The listing builds one solid part. Answer for the finished solid, in the listing's coordinates (mm). A direction names the side the tool comes from. Give positions to 0.01 mm unless a question says otherwise; leave off trailing zeros. Order: outer loops, then holes, each group sorted by start corner. A loop starts at its lowest first (then second) coordinate and runs counter-clockwise, first axis right, second up. Notation, with made-up numbers: (19, 2.5) - (64, 2.5) arc R15 cw to (64, 29.5) - close; hole circle Ø11 at (-33, -10.5). An arc over 180 degrees is marked (long way). Write each question's results on one line, items separated by ' | '. Start each with the question number.
1. Find the intervals of material crossed by L1, parallel to Z at x = -15.5, y = 0; L2, parallel to Y at x = -14, z = 1.5, in increasing order.
2. Which of the six approach directions +Z, -Z, +X, -X, +Y, -Y give full straight-line access (tool end or side, diameter ignored) to faces 4 (the face through (-61.5, 4, 12)), 5 (the face through (-76.014, -3.685, 11.701)), 6 (the face through (0, 0, 0))?
3. Section A-A (z = 0) is taken. Give the vertices of the cut face in (x, y).
4. Flat-ended cylindrical pins translate along their axes: pin 1 (5 mm diameter, centred on x = -77, y = 1.5, fed in from +Z); pin 2 (1 mm diameter, centred on x = -13.5, y = 1, fed in from +Z); pin 3 (3 mm diameter, centred on y = 5.5, z = 11, fed in from -X). Find the tip coordinate at first contact, or state that the pin passes through.
5. Section D-D (x = -120) is taken. Give the vertices of the cut face in (y, z).
6. Section C-C (x = -13) is taken. Give the vertices of the cut face in (y, z).
7. Determine the mould class of faces 1 (the face through (-64.035, 10.648, -13.887)), 2 (the face through (-80.56, -0.53, -11.99)), 3 (the face through (-8.16, 9.43, -2.09)) for opening direction X: released by +X, released by -X, zero draft, split by the parting line, or undercut.
from build123d import *

# Parameters (mm, degrees)
F2_SIZE2 = 2
F2_SIZE  = 2
F3_SIZE2 = 2.5
F3_SIZE  = 2.5


with BuildPart() as f1:
    # F0 (on Front) → F1 (revolve)
    with BuildSketch(Plane.XZ):
        with BuildLine():
            Line((-129.28461, 0), (0, 0))
            Line((0, 0), (0, 8.5))
            Line((0, 8.5), (-8, 8.5))
            Line((-8, 8.5), (-8, 12))
            Line((-8, 12), (-61.5, 12))
            Line((-61.5, 12), (-61.5, 17.5))
            Line((-61.5, 17.5), (-66.5, 17.5))
            Line((-66.5, 17.5), (-76.5, 12))
            Line((-76.5, 12), (-84.5, 12))
            ThreePointArc((-84.5, 12), (-111.496267, 23.18222), (-129.28461, 0))
        make_face()
    revolve(axis=Axis((-64.642305, 0, 0), (1, 0, 0)))

    # F2
    f2_edges = [f1.edges().sort_by_distance(p)[0] for p in [
        (0, 0, -8.5),
    ]]
    chamfer(f2_edges, length=F2_SIZE, length2=F2_SIZE2)

    # F3
    f3_edges = [f1.edges().sort_by_distance(p)[0] for p in [
        (-8, 0, -12),
    ]]
    chamfer(f3_edges, length=F3_SIZE, length2=F3_SIZE2)


solid = f1.part
Reported:
1) L1: -12 to 12 | L2: -11.91 to 11.91
2) face 4: +X | face 5: none | face 6: +Z, -Z, +X, +Y, -Y
3) outline: (-84.5, -12) - (-76.5, -12) - (-66.5, -17.5) - (-61.5, -17.5) - (-61.5, -12) - (-10.5, -12) - (-8, -9.5) - (-8, -8.5) - (-2, -8.5) - (0, -6.5) - (0, 6.5) - (-2, 8.5) - (-8, 8.5) - (-8, 9.5) - (-10.5, 12) - (-61.5, 12) - (-61.5, 17.5) - (-66.5, 17.5) - (-76.5, 12) - (-84.5, 12) arc R24 ccw (long way) to start
4) pin 1: z = 13.04 | pin 2: z = 11.99 | pin 3: x = -126.72
5) outline: circle Ø37.92 at (0, 0)
6) outline: circle Ø24 at (0, 0)
7) face 1: zero draft | face 2: undercut | face 3: released by +X
